For this review, use the dimensioned drawing (mm, ordinates from the lowest corner) and the shaded views. A direction names the side the tool comes from. Coordinates: 2 decimals unless noted, no trailing zeros. Write each loop counter-clockwise with the first axis right and the second up, starting at its lowest first coordinate (ties: lowest second). Pieces come first, ordered by that corner, then holes.
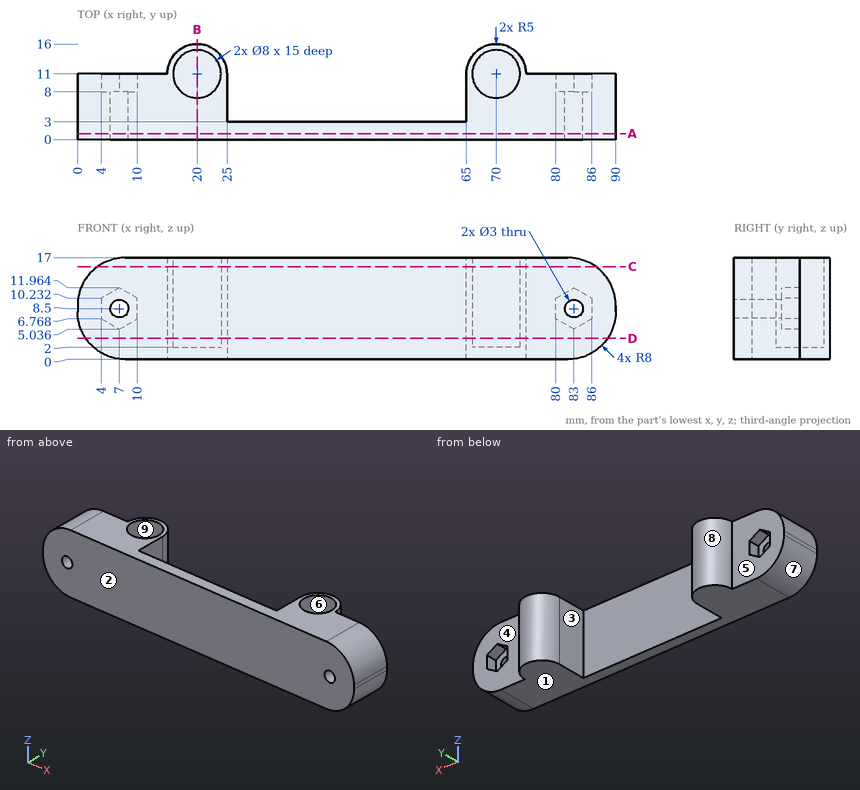
Item 1: Take a section at C-C, the plane z = 15.5. Write out the cut boundary in (x, y), plus the area to 3 significant figures.
Solved:
outline: (3.34, 0) - (86.66, 0) - (86.66, 11) - (75, 11) arc R5 ccw to (65, 11) - (65, 3) - (25, 3) - (25, 11) arc R5 ccw to (15, 11) - (3.34, 11) - close; hole circle Ø8 at (20, 11); hole circle Ø8 at (70, 11)
area: 575 mm2
Item 2: Take a section at B-B, the plane x = 20. Write out the cut boundary in (y, z), plus the area to 3 significant figures.
Solved:
outline: (0, 0) - (16, 0) - (16, 17) - (15, 17) - (15, 2) - (7, 2) - (7, 17) - (0, 17) - close
area: 152 mm2
Item 3: Machinability: for the marked faces 1, 2, 3, 4 and 5, which of the approach directions +Z, -Z, +X, -X, +Y, -Y give a long, thin tool a straight path to every point of the face, cutting with its end or side? Answer none if there is none.
Solved:
face 1: -Z, +X, -X, +Y, -Y
face 2: +Z, -Z, +X, -X, -Y
face 3: +Z, -Z, +Y
face 4: +Z, -Z, +X, +Y
face 5: +Z, -Z, -X, +Y
Item 4: For pin 1 (3 mm diameter, centred on x = 83.5, z = 7, fed in from +Y); pin 2 (6 mm diameter, centred on y = 5.5, z = 2, fed in from +X); pin 3 (1.5 mm diameter, centred on x = 60.5, z = 11, fed in from +Y), all flat-tipped, find the tip position at first contact; note any pin that passes through.
Solved:
pin 1: stops at y = 11
pin 2: stops at x = 89.42
pin 3: stops at y = 3
Item 5: To check wall thickness, follow line 1 along X through (y, z) = (4, 8.5); line 2 along X through (y, z) = (9.25, 4.5); line 3 along Y through (x, z) = (70, 11). State the ranges of each line that lie inside material, in increasing order.
Solved:
line 1: x = 0 to 5.5, 8.5 to 25, 65 to 81.5, 84.5 to 90
line 2: x = 0.81 to 16.4, 23.6 to 25, 65 to 66.4, 73.6 to 89.19
line 3: y = 0 to 7, 15 to 16
Item 6: Take a section at D-D, the plane z = 3.5. Write out the cut boundary in (x, y).
Solved:
outline: (1.39, 0) - (88.61, 0) - (88.61, 11) - (75, 11) arc R5 ccw to (65, 11) - (65, 3) - (25, 3) - (25, 11) arc R5 ccw to (15, 11) - (1.39, 11) - close; hole circle Ø8 at (20, 11); hole circle Ø8 at (70, 11)
Item 7: Mouldability with a two-part tool opening along Y and no side actions: class the marked faces 6, 7, 8 and 9 as pulls with the +Y half, pulls with the -Y half, needs draft (parallel to the pull), parting line crosses it, or undercut.
Solved:
face 6: undercut
face 7: needs draft
face 8: pulls with the +Y half
face 9: undercut
Item 8: Take a section at A-A, the plane y = 1. Write out the cut boundary in (x, z).
Solved:
outline: (0, 8) arc R8 ccw to (8, 0) - (82, 0) arc R8 ccw to (90, 8) - (90, 9) arc R8 ccw to (82, 17) - (8, 17) arc R8 ccw to (0, 9) - close; hole circle Ø3 at (7, 8.5); hole circle Ø3 at (83, 8.5)
